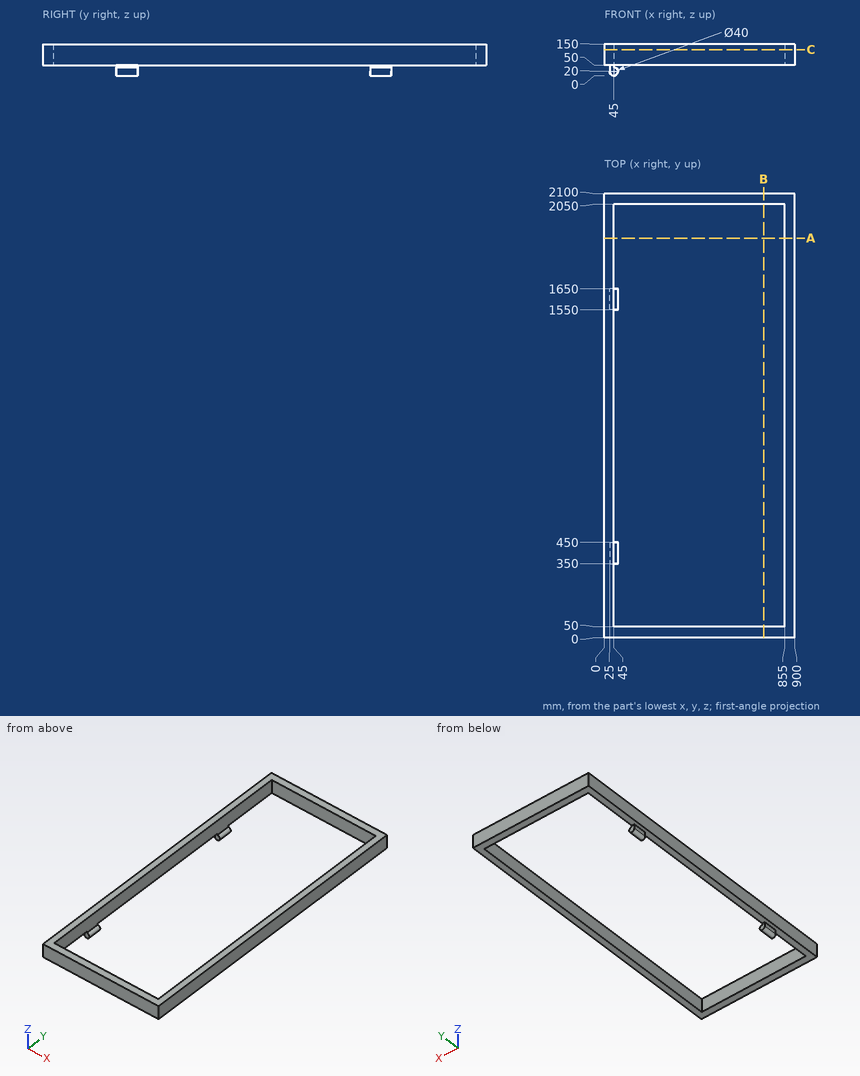
Geometry: see drawing. Coordinates: mm, zero at the bounding-box minimum. Coordinates: 2 decimals unless noted, no trailing zeros. Loops run counter-clockwise (first coordinate to the right, second up) from the corner with the lowest first, then second, coordinate; pieces in that order, holes last. Notation, with made-up numbers: (57.25, 74.5) -> (73.25, 74.5) arc R24 cw to (73.25, 91.5) -> close; hole circle Ø2 at (24.25, 55.5). An arc over 180 degrees is marked (long way). Write item = value, one per line. Start each with the question number.
Item 1: First-contact query: P1, Ø20, axis at x = 37, z = 25, coming from the +Y side; P2, Ø15, axis at y = 1596, z = 40.5, coming from the -X side. Flat tips, straight axial feed; report the tip coordinate or a pass-through.
Item 2: Cut plane A-A, the plane y = 1889.5. Return loops of the section in (x, z).
Item 3: Cut plane B-B, the plane x = 754. Return loops of the section in (y, z).
Item 4: Cut plane C-C, the plane z = 123. Return loops of the section in (x, y).
Item 5: Material intervals for line 1 (Y direction, x = 540, z = 68); line 2 (X direction, y = 622, z = 116.5), sorted ascending.
Ans:
q1.P1 = 1650
q1.P2 = 25
q2.outline = (0, 50) -> (45, 50) -> (45, 150) -> (0, 150) -> close; (855, 50) -> (900, 50) -> (900, 150) -> (855, 150) -> close
q3.outline = (0, 50) -> (50, 50) -> (50, 150) -> (0, 150) -> close; (2050, 50) -> (2100, 50) -> (2100, 150) -> (2050, 150) -> close
q4.outline = (0, 0) -> (900, 0) -> (900, 2100) -> (0, 2100) -> close; hole (45, 50) -> (855, 50) -> (855, 2050) -> (45, 2050) -> close
q5.line_1 = 0 to 50, 2050 to 2100
q5.line_2 = 0 to 45, 855 to 900
